```python
from build123d import *

# Parameters (mm, degrees)
SKETCH4_W                            = 30.48
SKETCH4_H                            = 2.54
F_3_0_213_DIAMETER_HOLE1_AT_2_COUNT  = 2
F_3_0_213_DIAMETER_HOLE1_AT_2_PITCH  = 63.5
F_3_0_213_DIAMETER_HOLE1_AT_3_COUNT  = 2
F_3_0_213_DIAMETER_HOLE1_AT_3_PITCH  = 32.870018728
F_3_0_213_DIAMETER_HOLE1_AT_4_COUNT  = 2
F_3_0_213_DIAMETER_HOLE1_AT_4_PITCH  = 63.5
F_3_0_213_DIAMETER_HOLE1_AT_5_COUNT  = 2
F_3_0_213_DIAMETER_HOLE1_AT_5_PITCH  = 89.802561211
F_3_0_213_DIAMETER_HOLE1_AT_6_COUNT  = 2
F_3_0_213_DIAMETER_HOLE1_AT_6_PITCH  = 109.985226281
F_3_0_213_DIAMETER_HOLE1_AT_7_COUNT  = 2
F_3_0_213_DIAMETER_HOLE1_AT_7_PITCH  = 122.672579939
F_3_0_213_DIAMETER_HOLE1_AT_8_COUNT  = 2
F_3_0_213_DIAMETER_HOLE1_AT_8_PITCH  = 127
F_3_0_213_DIAMETER_HOLE1_AT_9_COUNT  = 2
F_3_0_213_DIAMETER_HOLE1_AT_9_PITCH  = 122.672579939
F_3_0_213_DIAMETER_HOLE1_AT_10_COUNT = 2
F_3_0_213_DIAMETER_HOLE1_AT_10_PITCH = 109.985226281
F_3_0_213_DIAMETER_HOLE1_AT_11_COUNT = 2
F_3_0_213_DIAMETER_HOLE1_AT_11_PITCH = 89.802561211
F_3_0_213_DIAMETER_HOLE1_AT_12_COUNT = 2
F_3_0_213_DIAMETER_HOLE1_AT_12_PITCH = 63.5
F_3_0_213_DIAMETER_HOLE1_AT_13_COUNT = 2
F_3_0_213_DIAMETER_HOLE1_AT_13_PITCH = 32.870018728


with BuildPart() as part:
    # Sketch1 → Chamber (revolve)
    with BuildSketch(Plane(origin=(0, 0, 0), x_dir=(0, 0, -1), z_dir=(1, 0, 0))):
        Polygon((57.15, 6.35), (57.15, 114.3), (69.85, 114.3), (69.85, 120.65), (57.15, 120.65), (50.8, 120.65), (50.8, 114.3), (50.8, 6.35), (50.8, 0), (57.15, 0), (69.85, 0), (69.85, 6.35), align=None)
    revolve(axis=Axis((0, 0, 0), (0, 1, 0)))

    # Sketch4 → Turbulence Rings (revolve)
    with BuildSketch(Plane(origin=(0, 0, 0), x_dir=(0, 0, -1), z_dir=(1, 0, 0))):
        with Locations((35.56, 102.931657822)):
            Rectangle(SKETCH4_W, SKETCH4_H)
        with Locations((35.56, 17.718342178)):
            Rectangle(SKETCH4_W, SKETCH4_H)
    revolve(axis=Axis((0, 0, 0), (0, 1, 0)))

    # Sketch6 → #3 (0.213) Diameter Hole1 (revolve, cut)
    with BuildSketch(Plane(origin=(-54.99261314, 120.65, 31.75), x_dir=(0, 0, 1), z_dir=(1, 0, 0))):
        Polygon((0, 0), (0, 120.65), (3.3401, 120.65), (2.7051, 120.015), (2.7051, 0.635), (3.3401, 0), align=None)
    f_3_0_213_diameter_hole1 = revolve(axis=Axis((-54.99261314, 127, 31.75), (0, -1, 0)), mode=Mode.SUBTRACT)

    # #3 (0.213) Diameter Hole1 at 2: #3 (0.213) Diameter Hole1 ×2
    with Locations(*[Vector(0.866025404, 0, -0.5) * (i * F_3_0_213_DIAMETER_HOLE1_AT_2_PITCH) for i in range(1, F_3_0_213_DIAMETER_HOLE1_AT_2_COUNT)]):
        add(f_3_0_213_diameter_hole1, mode=Mode.SUBTRACT)

    # #3 (0.213) Diameter Hole1 at 3: #3 (0.213) Diameter Hole1 ×2
    with Locations(*[Vector(-0.258819045, 0, -0.965925826) * (i * F_3_0_213_DIAMETER_HOLE1_AT_3_PITCH) for i in range(1, F_3_0_213_DIAMETER_HOLE1_AT_3_COUNT)]):
        add(f_3_0_213_diameter_hole1, mode=Mode.SUBTRACT)

    # #3 (0.213) Diameter Hole1 at 4: #3 (0.213) Diameter Hole1 ×2
    with Locations(*[(0, 0, -i * F_3_0_213_DIAMETER_HOLE1_AT_4_PITCH) for i in range(1, F_3_0_213_DIAMETER_HOLE1_AT_4_COUNT)]):
        add(f_3_0_213_diameter_hole1, mode=Mode.SUBTRACT)

    # #3 (0.213) Diameter Hole1 at 5: #3 (0.213) Diameter Hole1 ×2
    with Locations(*[Vector(0.258819045, 0, -0.965925826) * (i * F_3_0_213_DIAMETER_HOLE1_AT_5_PITCH) for i in range(1, F_3_0_213_DIAMETER_HOLE1_AT_5_COUNT)]):
        add(f_3_0_213_diameter_hole1, mode=Mode.SUBTRACT)

    # #3 (0.213) Diameter Hole1 at 6: #3 (0.213) Diameter Hole1 ×2
    with Locations(*[Vector(0.5, 0, -0.866025404) * (i * F_3_0_213_DIAMETER_HOLE1_AT_6_PITCH) for i in range(1, F_3_0_213_DIAMETER_HOLE1_AT_6_COUNT)]):
        add(f_3_0_213_diameter_hole1, mode=Mode.SUBTRACT)

    # #3 (0.213) Diameter Hole1 at 7: #3 (0.213) Diameter Hole1 ×2
    with Locations(*[Vector(0.707106781, 0, -0.707106781) * (i * F_3_0_213_DIAMETER_HOLE1_AT_7_PITCH) for i in range(1, F_3_0_213_DIAMETER_HOLE1_AT_7_COUNT)]):
        add(f_3_0_213_diameter_hole1, mode=Mode.SUBTRACT)

    # #3 (0.213) Diameter Hole1 at 8: #3 (0.213) Diameter Hole1 ×2
    with Locations(*[Vector(0.866025404, 0, -0.5) * (i * F_3_0_213_DIAMETER_HOLE1_AT_8_PITCH) for i in range(1, F_3_0_213_DIAMETER_HOLE1_AT_8_COUNT)]):
        add(f_3_0_213_diameter_hole1, mode=Mode.SUBTRACT)

    # #3 (0.213) Diameter Hole1 at 9: #3 (0.213) Diameter Hole1 ×2
    with Locations(*[Vector(0.965925826, 0, -0.258819045) * (i * F_3_0_213_DIAMETER_HOLE1_AT_9_PITCH) for i in range(1, F_3_0_213_DIAMETER_HOLE1_AT_9_COUNT)]):
        add(f_3_0_213_diameter_hole1, mode=Mode.SUBTRACT)

    # #3 (0.213) Diameter Hole1 at 10: #3 (0.213) Diameter Hole1 ×2
    with Locations(*[(i * F_3_0_213_DIAMETER_HOLE1_AT_10_PITCH, 0, 0) for i in range(1, F_3_0_213_DIAMETER_HOLE1_AT_10_COUNT)]):
        add(f_3_0_213_diameter_hole1, mode=Mode.SUBTRACT)

    # #3 (0.213) Diameter Hole1 at 11: #3 (0.213) Diameter Hole1 ×2
    with Locations(*[Vector(0.965925826, 0, 0.258819045) * (i * F_3_0_213_DIAMETER_HOLE1_AT_11_PITCH) for i in range(1, F_3_0_213_DIAMETER_HOLE1_AT_11_COUNT)]):
        add(f_3_0_213_diameter_hole1, mode=Mode.SUBTRACT)

    # #3 (0.213) Diameter Hole1 at 12: #3 (0.213) Diameter Hole1 ×2
    with Locations(*[Vector(0.866025404, 0, 0.5) * (i * F_3_0_213_DIAMETER_HOLE1_AT_12_PITCH) for i in range(1, F_3_0_213_DIAMETER_HOLE1_AT_12_COUNT)]):
        add(f_3_0_213_diameter_hole1, mode=Mode.SUBTRACT)

    # #3 (0.213) Diameter Hole1 at 13: #3 (0.213) Diameter Hole1 ×2
    with Locations(*[Vector(0.707106781, 0, 0.707106781) * (i * F_3_0_213_DIAMETER_HOLE1_AT_13_PITCH) for i in range(1, F_3_0_213_DIAMETER_HOLE1_AT_13_COUNT)]):
        add(f_3_0_213_diameter_hole1, mode=Mode.SUBTRACT)


solid = part.part
```
Could you check a few things on this model? Use its own coordinates, in mm. A direction names the side the tool comes from. Round coordinates to 2 decimals unless told otherwise and drop trailing zeros. Write each loop counter-clockwise with the first axis right and the second up, starting at its lowest first coordinate (ties: lowest second). Pieces come first, ordered by that corner, then holes. Notation, with made-up numbers: M -37,11 L 15,11 A19 ccw 15,27 Z; hole C -31,-37.5 d5. An arc over 180 degrees is marked long. Answer in a Markdown table with one row per item. Add a question column.
Q1. Imagine slicing it at C-C (z = -23). Please give me the cut outline in (x, y), then the cut area to 3 significant figures.
Q2. Imagine slicing it at B-B (x = 47.5). Please give me the cut outline in (y, z), then the cut area to 3 significant figures.
Q3. Will these pins go through, and if not, where does the flat tip stop? pin 1 Ø4.5 at (x, z) = (54.99, -31.75) entering from -Y; pin 2 Ø5 at (x, y) = (36.5, 61) entering from +Z; pin 3 Ø12 at (y, z) = (17.5, 10) entering from +X; pin 4 Ø3 at (y, z) = (56.5, -48.5) entering from -X.
Q4. If we mould it in two halves opening along Y, with no side actions, what happens to faces 3 (the flat face through (-1, 101.662, 22)), 4 (the cylindrical face through (-60.86, 3.53, -0.59))? For each: +Y half, -Y half, draft (parallel to the pull), parting line (faces both ways), or undercut.
Q5. On a 3-axis mill with a long thin cutter (end or side, diameter ignored), from which of +Z, -Z, +X, -X, +Y, -Y can I reach the whole of each face in a straight line? I mean faces 1 (the cylindrical face through (33.396, 117.198, -57.139)), 2 (the cylindrical face through (-2.513, 61.081, 57.095)). Say none if no direction works.
Q6. If I drill on line 1 (X direction, y = 117.9, z = 0); line 2 (Y direction, x = -33.5, z = 13.5); line 3 (X direction, y = 89.5, z = 1), over which ranges is the centre line in solid material (lowest first)? Write a range as from..to.
Values:
| question | item | result |
|---|---|---|
| 1 | outline | M -65.95,0 L -45.3,0 L -45.3,16.45 L 45.3,16.45 L 45.3,0 L 65.95,0 L 65.95,6.35 L 52.32,6.35 L 52.32,114.3 L 65.95,114.3 L 65.95,120.65 L 45.3,120.65 L 45.3,104.2 L -45.3,104.2 L -45.3,120.65 L -65.95,120.65 L -65.95,114.3 L -52.32,114.3 L -52.32,6.35 L -65.95,6.35 Z; hole M -45.3,18.99 L 45.3,18.99 L 45.3,101.66 L -45.3,101.66 Z |
| 1 | area | 2,500 mm^2 |
| 2 | outline | M 0,-51.21 L 6.35,-51.21 L 6.35,-31.78 L 114.3,-31.78 L 114.3,-51.21 L 120.65,-51.21 L 120.65,-18.01 L 104.2,-18.01 L 104.2,18.01 L 120.65,18.01 L 120.65,51.21 L 114.3,51.21 L 114.3,31.78 L 6.35,31.78 L 6.35,51.21 L 0,51.21 L 0,18.01 L 16.45,18.01 L 16.45,-18.01 L 0,-18.01 Z; hole M 18.99,-18.01 L 101.66,-18.01 L 101.66,18.01 L 18.99,18.01 Z |
| 2 | area | 4,000 mm^2 |
| 3 | pin 1 | through |
| 3 | pin 2 | z = 45.94 |
| 3 | pin 3 | x = 57.01 |
| 3 | pin 4 | x = -32.51 |
| 4 | face 3 | undercut |
| 4 | face 4 | draft |
| 5 | face 1 | +Y, -Y |
| 5 | face 2 | none |
| 6 | line 1 | -69.85..-66.21, -60.79..-50.8, 50.8..60.79, 66.21..69.85 |
| 6 | line 2 | 16.45..18.99, 101.66..104.2 |
| 6 | line 3 | -57.14..-50.79, 50.79..57.14 |
